```python
from build123d import *

# Parameters (mm, degrees)
F0_R     = 14.2875
F1_DEPTH = 25.4
F2_DEPTH = 50.8


with BuildPart() as f1:
    # F0 (on Front) → F1 (new body)
    with BuildSketch(Plane.XZ):
        with BuildLine():
            ThreePointArc((7.2685239989, -27.6351078138), (22.6299436397, -17.4475292195), (28.575, 0))
            ThreePointArc((28.575, 0), (22.0602527934, 18.162485284), (5.4865750347, 28.0433257548))
            ThreePointArc((5.4865750347, 28.0433257548), (-28.5465468103, 1.2748687029), (2.9649285011, -28.4207639585))
            Line((2.9649285011, -28.4207639585), (7.2685239989, -27.6351078138))
        make_face()
        with BuildLine():
            ThreePointArc((-13.4703841816, 4.7625), (0, 14.2875), (13.4703841816, 4.7625))
            Line((13.4703841816, 4.7625), (19.05, 4.7625))
            Line((19.05, 4.7625), (19.05, -4.7625))
            Line((19.05, -4.7625), (13.4703841816, -4.7625))
            ThreePointArc((13.4703841816, -4.7625), (0, -14.2875), (-13.4703841816, -4.7625))
            Line((-13.4703841816, -4.7625), (-19.05, -4.7625))
            Line((-19.05, -4.7625), (-19.05, 4.7625))
            Line((-19.05, 4.7625), (-13.4703841816, 4.7625))
        make_face(mode=Mode.SUBTRACT)
        with BuildLine():
            ThreePointArc((5.4865750347, 28.0433257548), (22.0602527934, 18.162485284), (28.575, 0))
            ThreePointArc((28.575, 0), (22.6299436397, -17.4475292195), (7.2685239989, -27.6351078138))
            Line((7.2685239989, -27.6351078138), (54.3115272683, -19.0470273113))
            ThreePointArc((54.3115272683, -19.0470273113), (34.9605862818, -1.1638603674), (51.9860051328, 18.9458808034))
            Line((51.9860051328, 18.9458808034), (5.4865750347, 28.0433257548))
        make_face()
        with BuildLine():
            ThreePointArc((2.9649285011, -28.4207639585), (5.1317834533, -28.1104148598), (7.2685239989, -27.6351078138))
            Line((7.2685239989, -27.6351078138), (2.9649285011, -28.4207639585))
        make_face()
        with BuildLine():
            ThreePointArc((73.025, 0), (66.7227870193, 14.1561444649), (51.9860051328, 18.9458808034))
            ThreePointArc((51.9860051328, 18.9458808034), (34.9605862818, -1.1638603674), (54.3115272683, -19.0470273113))
            ThreePointArc((54.3115272683, -19.0470273113), (67.5638436679, -13.3508736706), (73.025, 0))
        make_face()
        with Locations((53.975, 0)):
            Circle(F0_R, mode=Mode.SUBTRACT)
    extrude(amount=F1_DEPTH)

    # F0 (on Front) → F2 (join)
    with BuildSketch(Plane.XZ):
        with BuildLine():
            ThreePointArc((7.2685239989, -27.6351078138), (22.6299436397, -17.4475292195), (28.575, 0))
            ThreePointArc((28.575, 0), (22.0602527934, 18.162485284), (5.4865750347, 28.0433257548))
            ThreePointArc((5.4865750347, 28.0433257548), (-28.5465468103, 1.2748687029), (2.9649285011, -28.4207639585))
            Line((2.9649285011, -28.4207639585), (7.2685239989, -27.6351078138))
        make_face()
        with BuildLine():
            ThreePointArc((-13.4703841816, 4.7625), (0, 14.2875), (13.4703841816, 4.7625))
            Line((13.4703841816, 4.7625), (19.05, 4.7625))
            Line((19.05, 4.7625), (19.05, -4.7625))
            Line((19.05, -4.7625), (13.4703841816, -4.7625))
            ThreePointArc((13.4703841816, -4.7625), (0, -14.2875), (-13.4703841816, -4.7625))
            Line((-13.4703841816, -4.7625), (-19.05, -4.7625))
            Line((-19.05, -4.7625), (-19.05, 4.7625))
            Line((-19.05, 4.7625), (-13.4703841816, 4.7625))
        make_face(mode=Mode.SUBTRACT)
        with BuildLine():
            ThreePointArc((-13.4703841816, -4.7625), (-14.2875, 0), (-13.4703841816, 4.7625))
            Line((-13.4703841816, 4.7625), (-19.05, 4.7625))
            Line((-19.05, 4.7625), (-19.05, -4.7625))
            Line((-19.05, -4.7625), (-13.4703841816, -4.7625))
        make_face()
    extrude(amount=F2_DEPTH)


solid = f1.part
```
Here's how the part is built. I have some questions about the finished solid (model axes, mm). A direction names the side the tool comes from. Round coordinates to 2 decimals unless told otherwise and drop trailing zeros. Loops run counter-clockwise (first coordinate to the right, second up) from the corner with the lowest first, then second, coordinate; pieces in that order, holes last. Notation, with made-up numbers: (6.25, 39) -> (12.25, 39) arc R23 ccw to (12.25, 70) -> close; hole circle Ø9 at (57, 40). An arc over 180 degrees is marked (long way). Answer as CSV lines item,"result". Start each with the question number.
1. Imagine slicing it at B-B on x = 0. Write out the boundary of the cut face in (y, z) (1 decimal), plus the area to 3 significant figures.
2. I need wall thicknesses on probe 1 along X at (y, z) = (-16, 2); probe 2 along Z at (x, y) = (0, -33) (1 decimal); probe 3 along Y at (x, z) = (69, 9). Which ranges of each line are inside material? Lowest first, please. Write a range as from..to.
3. If we mould it in two halves opening along X, with no side actions, what happens to faces 1 (the face through (39, -25.4, 2)), 2 (the face through (19.05, -25, 0)), 3 (the face through (5.087, -37.922, -28.033))? For each: pulls with the +X half, pulls with the -X half, needs draft (parallel to the pull), parting line crosses it, or undercut.
4. I'm going to push flat-ended pins straight in: P1, Ø10, axis at x = 7, y = -22, coming from the +Z side; P2, Ø1, axis at y = -44, z = 15, coming from the +X side; P3, Ø1, axis at x = 51, y = -14, coming from the +Z side; P4, Ø8, axis at x = -10, z = 4.5, coming from the +Y side. Where does each tip first touch, or does it pass through?
5. For faces 4 (the face through (22, 0, 0)), 5 (the face through (16, -25, -4.762)), which set-ups out of +Z, -Z, +X, -X, +Y, -Y let a thin tool reach every point of the face, with its end or its side?
6. Imagine slicing it at A-A on z = 0. State how many separate pieces and enclosed holes the cut face has, plus the area to 3 significant figures.
Solution:
1,outline,"(-50.8, -28.6) -> (0, -28.6) -> (0, -14.3) -> (-50.8, -14.3) -> close; (-50.8, 14.3) -> (0, 14.3) -> (0, 28.6) -> (-50.8, 28.6) -> close"
1,area,"1,450 mm²"
2,probe 1,"-28.5..-14.15, 19.05..39.83, 68.12..72.92"
2,probe 2,"-28.6..-14.3, 14.3..28.6"
2,probe 3,"-25.4..0"
3,face 1,"needs draft"
3,face 2,"undercut"
3,face 3,"pulls with the +X half"
4,P1,"z = 28.5"
4,P2,"x = 24.62"
4,P3,"z = 19.24"
4,P4,"y = 0"
5,face 4,"+Z, -Z, +X, -X, +Y"
5,face 5,"+Y, -Y"
6,separate pieces,"3"
6,enclosed holes,"0"
6,area,"1,610 mm²"
